Source: CAD feature listing. Evaluate the final solid. Frame: model axes, mm. Give positions to 0.01 mm unless a question says otherwise; leave off trailing zeros. Write each loop counter-clockwise with the first axis right and the second up, starting at its lowest first coordinate (ties: lowest second). Pieces come first, ordered by that corner, then holes.
```python
from build123d import *

# Parameters (mm, degrees)
EXTRUDE_1_DEPTH          = 123.83
CUT_EXTRUDE_1_DEPTH      = 10
PATTERN_CIRCULAR_4_COUNT = 8
SKETCH_5_R               = 7.9375
SKETCH_5_R_2             = 2.5
EXTRUDE_2_DEPTH          = 10
FILLET_1_R               = 7
SKETCH_7_R               = 1.5
CUT_EXTRUDE_3_DEPTH      = 40


with BuildPart() as part:
    # Sketch 1 → Extrude 1 (new body)
    with BuildSketch(Plane(origin=(0, 0, 0), x_dir=(1, 0, 0), z_dir=(0, 1, 0))):
        with BuildLine():
            Line((0, -11.906314203), (0, -7.9375))
            ThreePointArc((0, -7.9375), (3.037549744, -7.333293789), (5.612660076, -5.612660076))
            Line((5.612660076, -5.612660076), (8.419035512, -8.419035512))
            Line((8.419035512, -8.419035512), (0, -11.906314203))
        make_face()
    extrude_1 = extrude(amount=EXTRUDE_1_DEPTH)

    # Sketch 4 → Cut-Extrude 1 (cut, symmetric)
    with BuildSketch(Plane(origin=(0, 0, 0), x_dir=(0, 1, 0), z_dir=(0.923879533, 0, -0.382683432))):
        with BuildLine():
            Line((0, 13.154938161), (61.915, 13.154938161))
            Line((61.915, 13.154938161), (61.915, 11))
            add(Edge.make_bspline(
                [(61.915, 11), (41.306817411, 7.531903846), (20.665469899, 12.083633252), (0, 10.31)],
                knots=[0, 0, 0, 0, 1, 1, 1, 1], degree=3))
            Line((0, 10.31), (0, 13.154938161))
        make_face()
    cut_extrude_1 = extrude(amount=CUT_EXTRUDE_1_DEPTH, both=True, mode=Mode.SUBTRACT)

    # Pattern Circular 4: Extrude 1, Cut-Extrude 1 ×8 about axis
    pattern_circular_4_axis = Axis((0, 0, 0), (0, -1, 0))
    for i in range(1, PATTERN_CIRCULAR_4_COUNT):
        add(extrude_1.rotate(pattern_circular_4_axis, i * 360 / PATTERN_CIRCULAR_4_COUNT))
        add(cut_extrude_1.rotate(pattern_circular_4_axis, i * 360 / PATTERN_CIRCULAR_4_COUNT), mode=Mode.SUBTRACT)

    # Sketch 5 → Extrude 2 (add)
    with BuildSketch(Plane(origin=(0, 123.83, 0), x_dir=(1, 0, 0), z_dir=(0, 1, 0))):
        Circle(SKETCH_5_R)
        Circle(SKETCH_5_R_2, mode=Mode.SUBTRACT)
    extrude(amount=-EXTRUDE_2_DEPTH)

    # Fillet 1
    fillet_1_edges = [part.edges().sort_by_distance(p)[0] for p in [
        (10.162674858, 123.83, 4.209517756),
        (10.162674858, 123.83, -4.209517756),
        (4.209517756, 123.83, -10.162674858),
        (-4.209517756, 123.83, -10.162674858),
        (-10.162674858, 123.83, -4.209517756),
        (-10.162674858, 123.83, 4.209517756),
        (-4.209517756, 123.83, 10.162674858),
        (4.209517756, 123.83, 10.162674858),
    ]]
    fillet(fillet_1_edges, radius=FILLET_1_R)

    # Sketch 7 → Cut-Extrude 3 (cut)
    with BuildSketch(Plane(origin=(-4.209517756, 0, 10.162674858), x_dir=(0.923879533, 0, 0.382683432), z_dir=(-0.382683432, 0, 0.923879533))):
        with Locations((0, 61.915)):
            Circle(SKETCH_7_R)
    extrude(amount=-CUT_EXTRUDE_3_DEPTH, mode=Mode.SUBTRACT)


solid = part.part
```
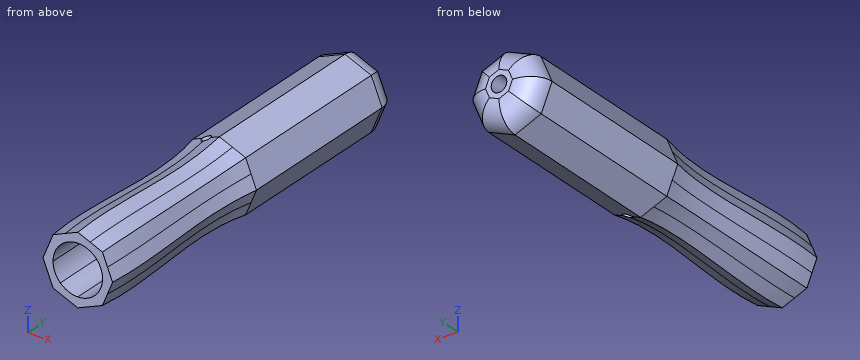
1. Line query: probe 1 along Y at (x, z) = (-2.5, -2.25); probe 2 along X at (y, z) = (112.5, -2.25); probe 3 along X at (y, z) = (93, 4.75). Output: solid intervals per line, ascending.
2. Section query A-A (y = 91). Return loops of the section in (x, z) (1 decimal).
3. Pin query (flat end, axial travel): P1, Ø2, axis at y = 84.5, z = -6.5, coming from the -X side; P2, Ø4, axis at x = -4, z = 1.5, coming from the -Y side; P3, Ø1, axis at x = -1, y = 90, coming from the +Z side. Return the tip coordinate at first contact, or that it passes through.
The answers:
1. probe 1: y = 113.83 to 123.83
1. probe 2: x = -10.97 to -7.61, 7.61 to 10.97
1. probe 3: x = -9.94 to -6.36, 6.36 to 9.94
2. outline: (-11.9, 0) - (-8.4, -8.4) - (0, -11.9) - (8.4, -8.4) - (11.9, 0) - (8.4, 8.4) - (0, 11.9) - (-8.4, 8.4) - close; hole circle Ø15.9 at (0, 0)
3. P1: stops at x = -9.63
3. P2: stops at y = 113.83
3. P3: stops at z = 11.7
